```python
from build123d import *

# Parameters (mm, degrees)
F0_W     = 627.888
F0_H     = 627.888
F1_DEPTH = 1016
F3_DEPTH = 209.296
F5_DEPTH = 209.296
F7_DEPTH = 209.296


with BuildPart() as f1:
    # F0 (on Top) → F1 (new body)
    with BuildSketch(Plane.XY):
        with Locations((152.424791, 157.284912)):
            Rectangle(F0_W, F0_H)
    extrude(amount=F1_DEPTH)

    # F2 (on face) → F3 (cut)
    with BuildSketch(Plane.YZ.offset(466.368791)):
        Polygon((-156.659088, 1016), (-156.659088, 177.8), (-125.163088, 177.8), (-125.163088, 228.6), (-93.667088, 228.6), (-93.667088, 279.4), (-62.171088, 279.4), (-62.171088, 330.2), (-30.675088, 330.2), (-30.675088, 381), (0.820912, 381), (0.820912, 431.8), (32.316912, 431.8), (32.316912, 482.6), (63.812912, 482.602637), (63.812912, 533.402637), (95.308912, 533.402637), (95.308912, 584.202637), (126.804912, 584.202637), (126.804912, 635.002637), (158.300912, 635.002637), (158.300912, 685.802637), (189.796912, 685.802637), (189.796912, 736.602637), (221.292912, 736.602637), (221.292912, 787.402637), (252.788912, 787.402637), (252.788912, 838.202637), (284.284912, 838.202637), (284.284912, 889.002637), (315.780912, 889.002637), (315.780912, 939.802637), (374.181002, 939.802637), (373.890931, 1016), align=None)
    extrude(amount=-F3_DEPTH, mode=Mode.SUBTRACT)

    # F4 (on face) → F5 (cut)
    with BuildSketch(Plane.YZ.offset(257.072791)):
        Polygon((-156.659088, 185.628965), (361.928195, 1016), (-156.659088, 1016), align=None)
    extrude(amount=-F5_DEPTH, mode=Mode.SUBTRACT)

    # F6 (on face) → F7 (cut)
    with BuildSketch(Plane(origin=(-161.519209, 0, 0), x_dir=(0, -1, 0), z_dir=(-1, 0, 0))):
        Polygon((156.659088, 1016), (-380.538228, 1016), (-380.538228, 911.203689), (-315.768228, 911.203689), (-315.768228, 860.403689), (-284.272228, 860.403689), (-284.272228, 809.603689), (-252.776228, 809.603689), (-252.776228, 758.803689), (-221.280228, 758.803689), (-221.280228, 708.003689), (-189.784228, 708.003689), (-189.784228, 657.203689), (-158.288228, 657.203689), (-158.288228, 606.403689), (-126.792228, 606.403689), (-126.792228, 555.603689), (-95.296228, 555.603689), (-95.296228, 517.449326), (-63.800228, 517.449326), (-63.800228, 482.611007), (-32.304228, 482.60837), (-32.304228, 431.80837), (-0.808228, 431.80837), (-0.808228, 381.00837), (30.687772, 381.00837), (30.687772, 330.20837), (62.183772, 330.20837), (62.183772, 279.40837), (93.679772, 279.40837), (93.679772, 228.60837), (125.175772, 228.60837), (125.175772, 177.80837), (156.659088, 177.80837), align=None)
    extrude(amount=-F7_DEPTH, mode=Mode.SUBTRACT)


solid = f1.part
```
Design review of the part built by this model. Coordinates are the model's own, in mm. A direction names the side the tool comes from. Give positions to 0.01 mm unless a question says otherwise; leave off trailing zeros. Write each loop counter-clockwise with the first axis right and the second up, starting at its lowest first coordinate (ties: lowest second). Pieces come first, ordered by that corner, then holes. Notation, with made-up numbers: (43, 48.25) - (49, 48.25) arc R12 cw to (49, 64.25) - close; hole circle Ø10 at (48.5, -33.75). An arc over 180 degrees is marked (long way). Return JSON: item names as keys, results as strings. Group by question number.
(1) We need section A-A, the plane z = 303.5. Give the boundary of the cut face in (x, y), then the cut area to 3 significant figures.
(2) To check wall thickness, follow probe 1 along Y at (x, z) = (-124.5, 455); probe 2 along Z at (x, y) = (-65.5, 29); probe 3 along Z at (x, y) = (352, 141). State the ranges of each line that lie inside material, in increasing order.
(3) We need section C-C, the plane y = 348. Give the boundary of the cut face in (x, z), then the cut area to 3 significant figures.
(4) Insertion check: pin 1 (4 mm diameter, centred on x = 399.5, y = 1.5, fed in from +Z); pin 2 (10 mm diameter, centred on x = -38, y = 136.5, fed in from +Z); pin 3 (6 mm diameter, centred on x = -56.5, y = 323, fed in from +Z); pin 4 (1 mm diameter, centred on x = 72.5, y = -90, fed in from -Z). Each pin has a flat end and moves straight along its axis. Give the tip position at first contact, or say it passes through.
(5) Machinability: for faces 1 (the flat face through (363, -110, 228.6)), 2 (the flat face through (148, 417, 1016)), 3 (the flat face through (-58, 206, 708.004)), which of the approach directions +Z, -Z, +X, -X, +Y, -Y give a long, thin tool a straight path to every point of the face, cutting with its end or side? Answer none if there is none.
(6) We need section B-B, the plane x = 110. Give the boundary of the cut face in (y, z).
Reported:
{
 "1": {"outline": "(-161.52, -62.18) - (47.78, -62.18) - (47.78, -83.05) - (257.07, -83.05) - (257.07, -62.17) - (466.37, -62.17) - (466.37, 471.23) - (-161.52, 471.23) - close", "area": "339,000 mm2"},
 "2": {"probe 1": "y = 32.3 to 471.23", "probe 2": "z = 0 to 431.81", "probe 3": "z = 0 to 635"},
 "3": {"outline": "(-161.52, 0) - (466.37, 0) - (466.37, 939.8) - (257.07, 939.8) - (257.07, 993.7) - (47.78, 993.7) - (47.78, 911.2) - (-161.52, 911.2) - close", "area": "595,000 mm2"},
 "4": {"pin 1": "stops at z = 431.8", "pin 2": "stops at z = 606.4", "pin 3": "stops at z = 911.2", "pin 4": "stops at z = 0"},
 "5": {"face 1": "+Z, +X, -Y", "face 2": "+Z, +X, -X, +Y, -Y", "face 3": "+Z, -X, -Y"},
 "6": {"outline": "(-156.66, 0) - (471.23, 0) - (471.23, 1016) - (361.93, 1016) - (-156.66, 185.63) - close"}
}
